```python
from build123d import *

# Parameters (mm, degrees)
IZIM1_W                     = 70
IZIM1_H                     = 40
Y_KSEKLIK_EKSTR_ZYON1_DEPTH = 40
BO_ALTMA2_T                 = 2
IZIM2_R                     = 2.5
IZIM2_R_2                   = 1
Y_KSEKLIK_EKSTR_ZYON2_DEPTH = 5
RADYUS2_R                   = 3
KES_EKSTR_ZYON1_DEPTH       = 5
KES_EKSTR_ZYON2_DEPTH       = 5
IZIM5_W                     = 3
IZIM5_H                     = 3
Y_KSEKLIK_EKSTR_ZYON3_DEPTH = 8
RADYUS3_R                   = 3
IZIM6_R                     = 1
KES_EKSTR_ZYON3_DEPTH       = 8
RADYUS4_R                   = 1.5


# Some blends are built 0.0001 mm under size
with BuildPart() as part:
    # Çizim1 → Yükseklik-Ekstrüzyon1 (new body)
    with BuildSketch(Plane.XY):
        Rectangle(IZIM1_W, IZIM1_H)
    extrude(amount=Y_KSEKLIK_EKSTR_ZYON1_DEPTH)

    # İç Boşaltma2
    bo_altma2_openings = [part.faces().sort_by_distance(p)[0] for p in [
        (0, 0, 40),
    ]]
    offset(amount=BO_ALTMA2_T, openings=bo_altma2_openings, kind=Kind.INTERSECTION)

    # Çizim2 → Yükseklik-Ekstrüzyon2 (add)
    # profile 1 of 4: a face of its own
    with BuildSketch(Plane.XY):
        with Locations((-30.8, 15.5)):
            Circle(IZIM2_R)
        with Locations((-30.8, 15.5)):
            Circle(IZIM2_R_2, mode=Mode.SUBTRACT)
    # profile 2 of 4: a face of its own
    with BuildSketch(Plane.XY):
        with Locations((-30.8, -15.5)):
            Circle(IZIM2_R)
        with Locations((-30.8, -15.5)):
            Circle(IZIM2_R_2, mode=Mode.SUBTRACT)
    # profile 3 of 4: a face of its own
    with BuildSketch(Plane.XY):
        with Locations((30.8, -15.5)):
            Circle(IZIM2_R)
        with Locations((30.8, -15.5)):
            Circle(IZIM2_R_2, mode=Mode.SUBTRACT)
    # profile 4 of 4: a face of its own
    with BuildSketch(Plane.XY):
        with Locations((30.8, 15.5)):
            Circle(IZIM2_R)
        with Locations((30.8, 15.5)):
            Circle(IZIM2_R_2, mode=Mode.SUBTRACT)
    extrude(amount=Y_KSEKLIK_EKSTR_ZYON2_DEPTH)

    # Radyus2
    radyus2_edges = [part.edges().sort_by_distance(p)[0] for p in [
        (0, -22, -2),
        (-37, 0, -2),
        (0, 22, -2),
        (37, 0, -2),
        (37, -22, 19),
        (-37, -22, 19),
        (-37, 22, 19),
        (37, 22, 19),
    ]]
    fillet(radyus2_edges, radius=RADYUS2_R)

    # Çizim3 → Kes-Ekstrüzyon1 (cut)
    with BuildSketch(Plane.ZY.offset(37)):
        Polygon((6.6, 3.36), (13.1, 3.36), (13.1, 0.86), (13.9, 0.86), (13.9, -2.64), (13.1, -2.64), (13.1, -5.14), (6.6, -5.14), align=None)
    extrude(amount=-KES_EKSTR_ZYON1_DEPTH, mode=Mode.SUBTRACT)

    # Çizim4 → Kes-Ekstrüzyon2 (cut)
    with BuildSketch(Plane(origin=(37, 0, 0), x_dir=(0, 0, -1), z_dir=(1, 0, 0))):
        Polygon((-13.1, -2.34), (-13.9, -2.34), (-13.9, 1.16), (-13.1, 1.16), (-13.1, 3.66), (-6.6, 3.66), (-6.6, -4.84), (-13.1, -4.84), align=None)
    extrude(amount=-KES_EKSTR_ZYON2_DEPTH, mode=Mode.SUBTRACT)

    # Çizim5 → Yükseklik-Ekstrüzyon3 (add)
    with BuildSketch(Plane.XY.offset(40)):
        with Locations((-33.5, 18.5)):
            Rectangle(IZIM5_W, IZIM5_H)
        with Locations((-33.5, -18.5)):
            Rectangle(IZIM5_W, IZIM5_H)
        with Locations((33.5, 18.5)):
            Rectangle(IZIM5_W, IZIM5_H)
        with Locations((33.5, -18.5)):
            Rectangle(IZIM5_W, IZIM5_H)
    extrude(amount=-Y_KSEKLIK_EKSTR_ZYON3_DEPTH)

    # Radyus3
    radyus3_edges = [part.edges().sort_by_distance(p)[0] for p in [
        (33.5, 20, 32),
        (35, 18.5, 32),
        (33.5, -20, 32),
        (35, -18.5, 32),
        (-35, -18.5, 32),
        (-33.5, -20, 32),
        (-33.5, 20, 32),
        (-35, 18.5, 32),
    ]]
    fillet(radyus3_edges, radius=RADYUS3_R - 0.0001)  # a hair under: the kernel refuses the full size

    # Çizim6 → Kes-Ekstrüzyon3 (cut)
    with BuildSketch(Plane.XY.offset(40)):
        with Locations((-34.5, 19.5)):
            Circle(IZIM6_R)
        with Locations((-34.5, -19.5)):
            Circle(IZIM6_R)
        with Locations((34.5, -19.5)):
            Circle(IZIM6_R)
        with Locations((34.5, 19.5)):
            Circle(IZIM6_R)
    extrude(amount=-KES_EKSTR_ZYON3_DEPTH, mode=Mode.SUBTRACT)

    # Radyus4
    # the kernel refuses this fillet: 1.5 mm, written as the material it takes off along each edge
    with BuildSketch(Plane(origin=(-32, -17, 43.75), x_dir=(-1, 0, 0), z_dir=(0, 0, -1)), Plane(origin=(-32, 17, 43.75), x_dir=(0, 1, 0), z_dir=(0, 0, -1))) as radyus4_piece_1:
        with BuildLine():
            CenterArc((RADYUS4_R, -RADYUS4_R), RADYUS4_R, 90, 90)
            Line((0, -RADYUS4_R), (0, 0))
            Line((0, 0), (RADYUS4_R, 0))
        make_face()
    extrude(amount=15.5, mode=Mode.SUBTRACT)
    with BuildSketch(Plane(origin=(32, -17, 43.75), x_dir=(1, 0, 0), z_dir=(0, 0, -1)), Plane(origin=(32, 17, 43.75), x_dir=(0, 1, 0), z_dir=(0, 0, -1))) as radyus4_piece_2:
        with BuildLine():
            CenterArc((RADYUS4_R, RADYUS4_R), RADYUS4_R, 180, 90)
            Line((0, RADYUS4_R), (0, 0))
            Line((0, 0), (RADYUS4_R, 0))
        make_face()
    extrude(amount=15.5, mode=Mode.SUBTRACT)


solid = part.part
```
CAD build for the part. Positions are in the model's coordinates, mm. A direction names the side the tool comes from. Coordinates: 2 decimals unless noted, no trailing zeros. Order: outer loops, then holes, each group sorted by start corner. A loop starts at its lowest first (then second) coordinate and runs counter-clockwise, first axis right, second up.
(1) Drill centre lines: L1, parallel to X at y = 17.5, z = 17; L2, parallel to Y at x = 30.8, z = 2.55; L3, parallel to Y at x = -25, z = 34.5. Where is each one in solid material? Low to high.
Solution:
L1: x = -37 to -35, 35 to 37
L2: y = -22 to -20, -18 to -16.5, -14.5 to -13, 13 to 14.5, 16.5 to 18, 20 to 22
L3: y = -22 to -20, 20 to 22
(2) Saw through at C-C, the plane x = 8. Write the cut outline in (y, z).
Solution:
outline: (-22, 1) arc R3 ccw to (-19, -2) - (19, -2) arc R3 ccw to (22, 1) - (22, 40) - (20, 40) - (20, 0) - (-20, 0) - (-20, 40) - (-22, 40) - close
(3) Pin check, flat tips, straight feed: pin 1 Ø4 at (x, y) = (-30, -15.5) entering from +Z; pin 2 Ø0.9 at (x, z) = (36, 13.5) entering from -Y; pin 3 Ø0.6 at (x, y) = (-30.5, 15.5) entering from +Z; pin 4 Ø3 at (x, y) = (34.5, -19.5) entering from +Z. Stop position of each tip, or through.
Solution:
pin 1: stops at z = 5
pin 2: stops at y = -21.57
pin 3: stops at z = 0
pin 4: stops at z = 40
(4) Saw through at B-B, the plane y = 0. Write the cut outline in (x, z), and give its area (3 significant figures).
Solution:
outline: (-37, 1) arc R3 ccw to (-34, -2) - (34, -2) arc R3 ccw to (37, 1) - (37, 6.6) - (35, 6.6) - (35, 0) - (-35, 0) - (-35, 6.6) - (-37, 6.6) - close; (-37, 13.9) - (-35, 13.9) - (-35, 40) - (-37, 40) - close; (35, 13.9) - (37, 13.9) - (37, 40) - (35, 40) - close
area: 275 mm2
(5) Saw through at A-A, the plane z = 2.5. Count the separate pieces of the cut face and the enclosed holes in it, and give its area (3 significant figures).
Solution:
separate pieces: 5
enclosed holes: 5
area: 514 mm2
(6) Saw through at D-D, the plane z = 25.5. Write the cut outline in (x, y).
Solution:
outline: (-37, -19) arc R3 ccw to (-34, -22) - (34, -22) arc R3 ccw to (37, -19) - (37, 19) arc R3 ccw to (34, 22) - (-34, 22) arc R3 ccw to (-37, 19) - close; hole (-35, -20) - (35, -20) - (35, 20) - (-35, 20) - close
(7) Mould opens along Y. For faces 3 (the face through (31, 16, 0)), 4 (the face through (0, -22, 20)), 5 (the face through (37, 0, 20)) say: released by +Y, released by -Y, zero draft, split by the parting line, or undercut.
Solution:
face 3: undercut
face 4: released by -Y
face 5: zero draft
(8) Which spindle directions (+Z, -Z, +X, -X, +Y, -Y) get a long thin tool onto all of the face, cutting with end or side? Do faces 1 (the face through (36, -4.84, 10)), 2 (the face through (-32.45, -17.43, 35.86)). Say none if no direction does.
Solution:
face 1: +X, -X
face 2: +Z
